CAD build for the part. Positions are in the model's coordinates, mm. A direction names the side the tool comes from. Give positions to 0.01 mm unless a question says otherwise; leave off trailing zeros. Write each loop counter-clockwise with the first axis right and the second up, starting at its lowest first coordinate (ties: lowest second). Pieces come first, ordered by that corner, then holes. Notation, with made-up numbers: (36.25, 71.5) -> (93.25, 71.5) arc R13 cw to (93.25, 91.5) -> close; hole circle Ø10 at (-35, 81.25). An arc over 180 degrees is marked (long way). Answer as a JSON object with one key per item and string values.
```python
from build123d import *

# Parameters (mm, degrees)
EXTRUDE1_START = -1
EXTRUDE1_DEPTH = 2.03
EXTRUDE2_DEPTH = 4.06
SKETCH4_R      = 5.08
SKETCH4_R_2    = 2.6035
SKETCH4_R_3    = 0.97028
EXTRUDE3_DEPTH = 33.328789028
FILLET1_R      = 3.175


with BuildPart() as part:
    # Sketch1 → Extrude1 (new body)
    with BuildSketch(Plane.XY.offset(EXTRUDE1_START)):
        Polygon((0, 19.05), (0, 0), (25.4, 0), (25.4, 5.851775032), (2.540003786, 19.05), align=None)
    extrude(amount=-EXTRUDE1_DEPTH)

    # Sketch2 → Extrude2 (add)
    with BuildSketch(Plane(origin=(0, 0, -3.03), x_dir=(-1, 0, 0), z_dir=(0, 0, -1))):
        with BuildLine():
            Line((-11.896721187, 0), (-25.4, 0))
            Line((-25.4, 0), (-25.4, 5.851775032))
            Line((-25.4, 5.851775032), (-15.066541319, 11.817800183))
            ThreePointArc((-15.066541319, 11.817800183), (-14.71969706, 5.576820867), (-11.896721187, 0))
        make_face()
    extrude(amount=EXTRUDE2_DEPTH)

    # Sketch4 → Extrude3 (cut, through all)
    with BuildSketch(Plane(origin=(0, 0, -7.09), x_dir=(-1, 0, 0), z_dir=(0, 0, -1))):
        with Locations((0, 9.525)):
            Circle(SKETCH4_R)
        with Locations(Location((-19.05, 4.7625, 0), (0, 0, 180))):
            Circle(SKETCH4_R_2)
        with Locations(Location((-7.4422, 9.525, 0), (0, 0, 180))):
            Circle(SKETCH4_R_3)
    extrude(amount=-EXTRUDE3_DEPTH, mode=Mode.SUBTRACT)

    # Fillet1
    fillet1_edges = [part.edges().sort_by_distance(p)[0] for p in [
        (2.540003786, 19.05, -2.015),
        (25.4, 5.851775032, -4.045),
        (25.4, 0, -4.045),
    ]]
    fillet(fillet1_edges, radius=FILLET1_R)

    # Mirror1: part across plane


with BuildPart() as part_1:
    add(part.part)
    add(part.part.mirror(Plane(origin=(0, 19.05, -3.03), x_dir=(0, 0, 1), z_dir=(-1, 0, 0))))


solid = part_1.part
```
1) Slice it at D-D (y = 6). List the corners of the cut face in (x, z), then the cut area to 3 significant figures.
Model answer:
{"outline": "(-24.71, -7.09) -> (-21.34, -7.09) -> (-21.34, -1) -> (-24.71, -1) -> close; (-16.76, -7.09) -> (-14.83, -7.09) -> (-14.83, -3.03) -> (-3.66, -3.03) -> (-3.66, -1) -> (-16.76, -1) -> close; (3.66, -3.03) -> (14.83, -3.03) -> (14.83, -7.09) -> (16.76, -7.09) -> (16.76, -1) -> (3.66, -1) -> close; (21.34, -7.09) -> (24.71, -7.09) -> (24.71, -1) -> (21.34, -1) -> close", "area": "110 mm2"}
2) Pin check, flat tips, straight feed: pin 1 (1.7 mm diameter, centred on x = 7.44, y = 9.52, fed in from -Z); pin 2 (10 mm diameter, centred on x = 5, y = 10, fed in from -Z); pin 3 (2 mm diameter, centred on y = 10, z = -2, fed in from -X). Stop position of each tip, or through.
Model answer:
{"pin 1": "passes through", "pin 2": "stops at z = -3.03", "pin 3": "stops at x = -19.95"}
3) Slice it at B-B (x = 0). List the corners of the cut face in (y, z) (3 decimals).
Model answer:
{"outline": "(0, -3.03) -> (4.445, -3.03) -> (4.445, -1) -> (0, -1) -> close; (14.605, -3.03) -> (19.05, -3.03) -> (19.05, -1) -> (14.605, -1) -> close"}
4) Slice it at A-A (z = -6.5). State how many separate pieces and enclosed holes the cut face has, then the cut area to 3 significant figures.
Model answer:
{"separate pieces": "2", "enclosed holes": "2", "area": "151 mm2"}
5) Wall check: probe 1 along X at (y, z) = (4.5, -3.25); probe 2 along X at (y, z) = (3, -2); probe 3 along Y at (x, z) = (0, -2.4) (3 decimals). Give the ranges that are in metal, low to high.
Model answer:
{"probe 1": "x = -25.36 to -21.64, -16.46 to -14.39, 14.39 to 16.46, 21.64 to 25.36", "probe 2": "x = -25.4 to -20.97, -17.13 to 17.13, 20.97 to 25.4", "probe 3": "y = 0 to 4.445, 14.605 to 19.05"}
6) 3-axis set-ups, long thin cutter, end or side, ignore diameter. For faces 1 (the flat face through (25.4, 3.6, -4)), 2 (the cylindrical face through (-14.74, 5.66, -5.03)): which of +Z, -Z, +X, -X, +Y, -Y reach the whole face in a straight line?
Model answer:
{"face 1": "+Z, -Z, +X, +Y, -Y", "face 2": "-Z"}
7) Mould opens along X. For faces 3 (the flat face through (0.3, 0, -2.6)), 4 (the cylindrical face through (-24.45, 0.91, -4)), 5 (the cylindrical face through (24.45, 0.91, -4)), 6 (the cylindrical face through (14.74, 5.66, -5.03)) say: released by +X, released by -X, zero draft, split by the parting line, or undercut.
Model answer:
{"face 3": "zero draft", "face 4": "released by -X", "face 5": "released by +X", "face 6": "undercut"}
